Design review of the part built by this model. Coordinates are the model's own, in mm. A direction names the side the tool comes from. Coordinates: 2 decimals unless noted, no trailing zeros. Order: outer loops, then holes, each group sorted by start corner. A loop starts at its lowest first (then second) coordinate and runs counter-clockwise, first axis right, second up. Notation, with made-up numbers: (-33, -16) -> (3, -16) arc R22 cw to (3, 21) -> close; hole circle Ø10 at (-19, 0.25). An arc over 180 degrees is marked (long way). Use a Markdown table: item, result. Add a question column.
Q1. Wall thickness on probe 1 along X at (y, z) = (-67.5, -20); probe 2 along Z at (x, y) = (-1.5, -43): over which ranges is each line inside the solid? List them lowest first.
Q2. Machinability: for faces 1 (the face through (-11, -82, -42.235)), 2 (the face through (8.982, -67, -18)), 3 (the face through (-17.09, -74.7, -35.97)), which of the approach directions +Z, -Z, +X, -X, +Y, -Y give a long, thin tool a straight path to every point of the face, cutting with its end or side? Answer none if there is none.
Q3. Add section B-B (y = -106). State the section outline as (x, z) points, then the cut area to 3 significant figures.
Q4. The part is to be moulded in two halves that separate along X. For faces 4 (the face through (-48.168, -67, -26)), 5 (the face through (-12, -71, -29.535)), 6 (the face through (28.032, -67, -27)), say which applies: pulls with the +X half, pulls with the -X half, needs draft (parallel to the pull), parting line crosses it, or undercut.
Q5. Insertion check: pin 1 (10 mm diameter, centred on x = -10.07, y = -68.26, fed in from +Z); pin 2 (11.5 mm diameter, centred on x = -10.07, y = -68.26, fed in from -Z). Each pin has a flat end and moves straight along its axis. Give the tip position at first contact, or say it passes through.
Q6. Add section C-C (x = 1). State the section outline as (y, z) points (3 decimals), then the cut area to 3 significant figures.
Q7. Add section A-A (z = -23). State the section outline as (x, y) points (3 decimals).
from build123d import *

# Parameters (mm, degrees)
F1_DEPTH = 136.525
F2_R     = 3.175
F3_DEPTH = 6.35
F5_R     = 9.525
F6_DEPTH = 12.7
F4_R     = 3.175
F7_DEPTH = 25.4


with BuildPart() as f1:
    # F0 (on Front) → F1 (new body)
    with BuildSketch(Plane.XZ):
        Polygon((-48.16837, -10.484883), (-48.16837, -42.234883), (28.03163, -42.234883), (28.03163, -10.484883), (8.98163, -10.484883), (8.98163, -25.545781), (-29.11837, -25.545781), (-29.11837, -10.484883), align=None)
    extrude(amount=F1_DEPTH)

    # F2 (on face) → F3 (join)
    with BuildSketch(Plane.XY.offset(-25.545781)):
        with Locations((-10.06837, -68.2625)):
            Circle(F2_R)
    extrude(amount=-F3_DEPTH)

    # F5 (on face) → F6 (cut)
    with BuildSketch(Plane(origin=(0, 0, -42.234883), x_dir=(1, 0, 0), z_dir=(0, 0, -1))):
        with Locations((-10.06837, 68.2625)):
            Circle(F5_R)
    extrude(amount=-F6_DEPTH, mode=Mode.SUBTRACT)

    # F4 (on face) → F7 (cut)
    with BuildSketch(Plane.XY.offset(-25.545781)):
        with Locations((-10.06837, -68.2625)):
            Circle(F4_R)
    extrude(amount=-F7_DEPTH, mode=Mode.SUBTRACT)


solid = f1.part
Established:
| question | item | result |
|---|---|---|
| 1 | probe 1 | -48.17 to -29.12, 8.98 to 28.03 |
| 1 | probe 2 | -42.23 to -25.55 |
| 2 | face 1 | -Z, +X, -X, +Y, -Y |
| 2 | face 2 | +Z, +Y, -Y |
| 2 | face 3 | -Z |
| 3 | outline | (-48.17, -42.23) -> (28.03, -42.23) -> (28.03, -10.48) -> (8.98, -10.48) -> (8.98, -25.55) -> (-29.12, -25.55) -> (-29.12, -10.48) -> (-48.17, -10.48) -> close |
| 3 | area | 1,850 mm^2 |
| 4 | face 4 | pulls with the -X half |
| 4 | face 5 | undercut |
| 4 | face 6 | pulls with the +X half |
| 5 | pin 1 | z = -25.55 |
| 5 | pin 2 | z = -29.53 |
| 6 | outline | (-136.525, -42.235) -> (0, -42.235) -> (0, -25.546) -> (-136.525, -25.546) -> close |
| 6 | area | 2,280 mm^2 |
| 7 | outline | (-48.168, -136.525) -> (-29.118, -136.525) -> (-29.118, 0) -> (-48.168, 0) -> close; (8.982, -136.525) -> (28.032, -136.525) -> (28.032, 0) -> (8.982, 0) -> close |
